Autodesk Inventor part; units mm, degrees
ref_plane "YZ Plane" through (0, 0, 0) normal (1, 0, 0) x (0, 1, 0)
ref_plane "XZ Plane" through (0, 0, 0) normal (0, 1, 0) x (-1, 0, 0)
ref_plane "XY Plane" through (0, 0, 0) normal (0, 0, 1) x (1, 0, 0)
sketch "Sketch1" plane through (0, 0, 0) normal (0, 0, 1) x (1, 0, 0)
  line L0 (0, 0) -> (119.6, 0)
  line L1 (119.6, 0) -> (119.6, 150)
  line L2 (119.6, 150) -> (0, 150)
  line L3 (0, 150) -> (0, 0)
  dimension "d0" = 119.6
  dimension "d1" = 150
sketch "Sketch2" plane through (0, 0, 0) normal (1, 0, 0) x (0, 1, 0)
  circle A0 centre (0, 0) radius 12.5
  circle A1 centre (0, 0) radius 6.125
  line L0 (-12.5, 0) -> (12.5, 0)
  line L1 (12.5, 0) -> (12.5, 12.5)
  line L2 (12.5, 12.5) -> (-12.5, 12.5)
  line L3 (-12.5, 12.5) -> (-12.5, 0)
  circle A2 centre (150, 0) radius 12.5
  circle A3 centre (150, 0) radius 6.125
  line L4 (137.5, 0) -> (162.5, 0)
  line L5 (162.5, 0) -> (162.5, 12.5)
  line L6 (162.5, 12.5) -> (137.5, 12.5)
  line L7 (137.5, 12.5) -> (137.5, 0)
  line L8 (-12.5, 12.5) -> (-17.5, 12.5)
  line L9 (-17.5, 12.5) -> (-17.5, 0)
  line L10 (-17.5, 0) -> (-12.5, 0)
  line L11 (-12.5, 0) -> (-12.5, 12.5)
  line L12 (12.5, 12.5) -> (17.5, 12.5)
  line L13 (17.5, 12.5) -> (17.5, 0)
  line L14 (17.5, 0) -> (12.5, 0)
  line L15 (12.5, 0) -> (12.5, 12.5)
  point P0 (6.125, 0)
  point P1 (-6.125, 0)
  point P2 (150, 0)
  point P3 (12.5, 0)
  dimension "d2" = 25
  dimension "d3" = 12.25
  dimension "d6" = 5
  dimension "d7" = 5
  dimension "d8" = 35
extrude "Extrusion1" add sketch "Sketch2" along normal up to surface (119.6 mm away) contours L3 L2 A0 | A0 L0 A1 | L10 L9 L8 L3 | A0 L2 L1 | L1 L12 L13 L14 | A1 L0 picked at (10.2705, 0.9272) picked at (1.5282, 2.3311)
ref_plane "Work Plane1" through (59.8, 0, 0) normal (-1, 0, 0) x (0, 0, 1)
sketch "Sketch3" plane through (0, -17.5, 0) normal (0, -1, 0) x (1, 0, 0)
  line L0 (0, 12.5) -> (119.6, 12.5)
  line L1 (102.1, 12.5) -> (137.1, 12.5)
  line L2 (137.1, 12.5) -> (137.1, 0)
  line L3 (137.1, 0) -> (102.1, 0)
  line L4 (102.1, 0) -> (102.1, 12.5)
  line L5 (119.6, 12.5) -> (119.6, 0)
  circle A0 centre (119.6, 0) radius 8.925
  point P0 (0, 0)
  point P1 (119.6, 12.5)
  point P2 (128.525, 0)
  point P3 (110.675, 0)
  dimension "d9" = 35
  dimension "d33" = 17.85
extrude "Extrusion2" add sketch "Sketch3" against normal blind 55 contours L0 L5 A0 L3 L4 | L1 L2 L3 A0 L5 | A0 L3 L5 | L5 L3 A0
extrude "Extrusion4" cut sketch "Sketch3" along normal through all both and the other way through all contours A0 L3 L5 | L5 L3 A0
extrude "Extrusion3" cut sketch "Sketch2" along normal up to surface (119.6 mm away) contours A1 L0 picked at (1.5282, 2.3311)
mirror "Mirror1" about plane through (59.8, 0, 0) normal (-1, 0, 0) of "Extrusion2", "Extrusion4", "Extrusion3"
sketch "Sketch4" plane through (102.1, 17.5, 12.5) normal (0, 0, 1) x (1, 0, 0)
  line L0 (-119.6, -35) -> (35, -35)
  line L1 (0, 20) -> (35, 20)
  line L2 (0, 0) -> (0, 20)
  line L3 (-84.6, 0) -> (0, 0)
  line L4 (-84.6, 0) -> (-84.6, 20)
  line L5 (-84.6, 20) -> (-119.6, 20)
  line L6 (35, -35) -> (35, 20)
  line L7 (-119.6, -35) -> (-119.6, 20)
  point P0 (-102.1, -17.5)
extrude "Extrusion5" add sketch "Sketch4" along normal blind 5
sketch "Sketch5" plane through (102.1, 17.5, 0) normal (0, 0, -1) x (-1, 0, 0)
  circle A0 centre (16.425, -6.375) radius 2
  line L0 (-8.575, -11.375) -> (93.175, -11.375)
  line L1 (-8.575, 20) -> (-8.575, -11.375)
  circle A1 centre (65.675, -6.375) radius 2
  circle A2 centre (16.425, -28.625) radius 2
  circle A3 centre (65.675, -28.625) radius 2
  line L2 (93.175, -35) -> (93.175, -23.625)
  line L3 (93.175, -23.625) -> (-8.575, -23.625)
  circle A4 centre (-30, -17.5) radius 2
  circle A5 centre (117.6, -17.5) radius 2
  line L4 (-35, -35) -> (-35, 20)
  line L5 (119.6, -35) -> (119.6, 20)
  line L6 (16.425, -6.375) -> (16.425, -28.625) construction
  point P0 (102.1, -17.5)
  point P1 (16.425, -17.5)
  dimension "d18" = 4
  dimension "d19" = 5
  dimension "d20" = 25
  dimension "d23" = 49.25
  dimension "d26" = 22.25
  dimension "d29" = 27.5
  dimension "d30" = 5
  dimension "d38" = 5
  dimension "d39" = 2
extrude "Extrusion6" cut sketch "Sketch5" against normal blind 13.5
sketch "Sketch6" plane through (0, 37.5, 0) normal (0, 1, 0) x (1, 0, 0)
  circle A0 centre (0, 0) radius 12.325
  line L0 (-17.5, 0) -> (-17.5, -17.5)
  line L1 (-17.5, -17.5) -> (-21, -17.5)
  line L2 (-21, -17.5) -> (-21, 0)
  line L3 (-21, 0) -> (-17.5, 0)
  line L4 (-17.5, 0) -> (-17.5, -17.5)
  line L5 (-17.5, 0) -> (-8.925, 0)
  dimension "d34" = 24.65
  dimension "d40" = 3.5
extrude "Extrusion7" cut sketch "Sketch6" against normal through all contours A0
extrude "Extrusion8" add sketch "Sketch6" against normal up to surface (55 mm away) contours L0 L1 L2 L3
fillet "Fillet1" radius 2 8 edges at (102.1, 17.5, 8.75) (17.5, 17.5, 8.75) (17.5, 37.5, 8.75) (102.1, 37.5, 8.75) (137.1, 37.5, 8.75) (137.1, -17.5, 8.75) (-21, 37.5, 8.75) (-21, -17.5, 8.75)
sketch "Sketch7" plane through (-21, -15.5, 17.5) normal (-1, 0, 0) x (0, 0, 1)
  circle A0 centre (-3.7125, 10) radius 2
  line L0 (0, 51) -> (0, 0)
  line L1 (-17.5, -2) -> (0, -2)
  circle A1 centre (-3.7125, 47.75) radius 2
  point P0 (-17.5, 15.5)
  dimension "d43" = 4
  dimension "d44" = 3.7125
  dimension "d45" = 12
  dimension "d49" = 37.75
extrude "Extrusion9" cut sketch "Sketch7" against normal blind 5
extrude "Extrusion10" cut sketch "Sketch7" along normal blind 5 from surface at -158.1
equation "\"d7\" = d6"
equation "\"d9\" = d8"
properties part number "BottomBase"
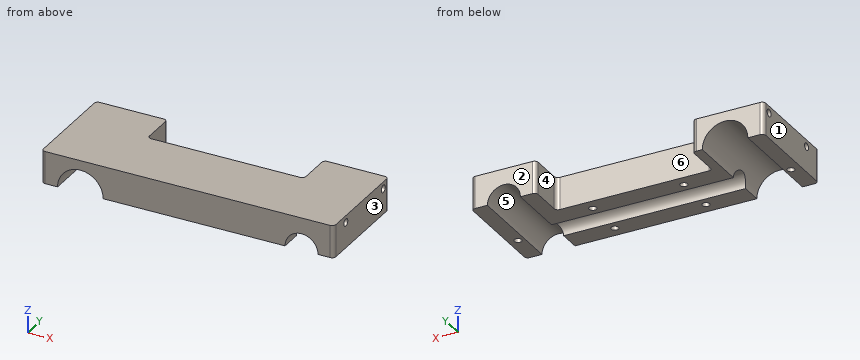
Input: part model. Units: mm. Frame: model coordinates. Face numbers are marked on the shaded views. A direction names the side the tool comes from. Give positions to 0.01 mm unless a question says otherwise; leave off trailing zeros. Order: outer loops, then holes, each group sorted by start corner. A loop starts at its lowest first (then second) coordinate and runs counter-clockwise, first axis right, second up. Notation, with made-up numbers: M 34,25 L 48,25 A34 ccw 48,55 Z; hole C 62.5,72 d11. An arc over 180 degrees is marked long. One line per question, with ' | ' between items. Start each with the question number.
1. Section query A-A (z = 4.75). Count the separate pieces of the cut face and the enclosed holes in it, and give its area (3 significant figures).
2. Access query for the marked faces 5 and 6. Directions: +Z, -Z, +X, -X, +Y, -Y. A direction counts if a zero-diameter tool reaches every point of the face in a straight line with its end or side. Return the directions, or none.
3. Section query D-D (x = 42.5). Return the cut outline in (y, z) (3 decimals), and give its area (3 significant figures).
4. Section query C-C (y = 25). Return the cut outline in (x, z) (3 decimals), and give its area (3 significant figures).
5. Pull-direction query (X, two-part tool) for the marked faces 1, 2, 3 and 4; classes: released by +X, released by -X, zero draft, split by the parting line, or undercut.
6. Material intervals for probe 1 along X at (y, z) = (7.5, 5.25); probe 2 along X at (y, z) = (28, 7); probe 3 along X at (y, z) = (10, 5.5), sorted ascending. Write a range as [from, to].
7. First-contact query: pin 1 Ø4.5 at (x, y) = (36.5, -11) entering from -Z; pin 2 Ø3 at (x, y) = (85.675, -11.125) entering from -Z; pin 3 Ø2.5 at (y, z) = (-5.5, 13.79) entering from +X; pin 4 Ø2.5 at (y, z) = (32.25, 13.79) entering from -X. Flat tips, straight axial feed; report the tip coordinate or a pass-through.
Here are the results:
1) separate pieces: 4 | enclosed holes: 6 | area: 4,060 mm²
2) face 5: -Z, +Y, -Y | face 6: +Z, -Z, +Y
3) outline: M -17.5,0 L -6.125,0 A6.125 cw 6.125,0 L 17.5,0 L 17.5,17.5 L -17.5,17.5 Z | area: 554 mm²
4) outline: M -21,0 L -12.325,0 A12.325 cw 12.325,0 L 17.5,0 L 17.5,17.5 L -21,17.5 Z; M 102.1,0 L 110.675,0 A8.925 cw 128.525,0 L 137.1,0 L 137.1,17.5 L 102.1,17.5 Z | area: 923 mm²
5) face 1: released by -X | face 2: zero draft | face 3: released by +X | face 4: undercut
6) probe 1: [-21, -11.15], [11.15, 112.38], [126.82, 137.1] | probe 2: [-21, -10.14], [10.14, 17.5], [102.1, 114.06], [125.14, 137.1] | probe 3: [-21, -11.03], [11.03, 34.77], [38.08, 84.02], [87.33, 112.57], [126.63, 137.1]
7) pin 1: z = 0 | pin 2: z = 13.5 | pin 3: x = 132.1 | pin 4: x = -16
